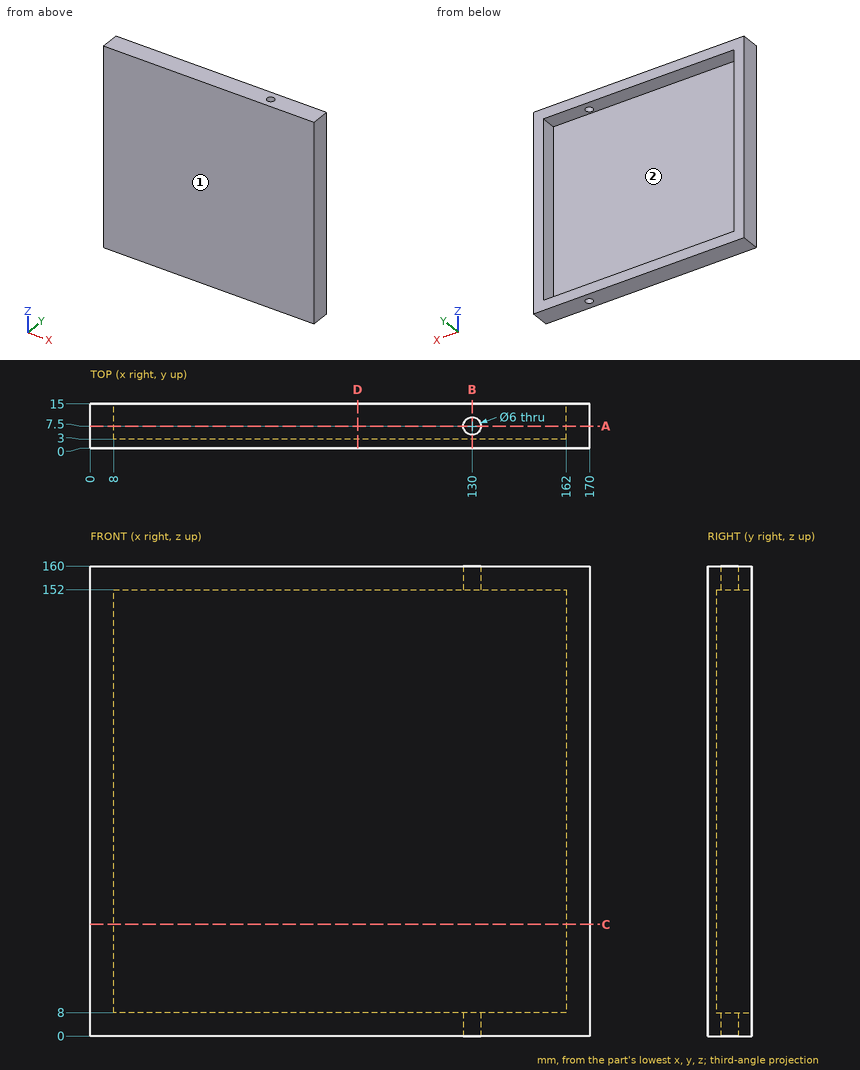
Design review of the part shown in the three views and the two pictorial views. Dimensions are in mm from the part's minimum x, y and z. Round coordinates to 2 decimals unless told otherwise and drop trailing zeros. Write each loop counter-clockwise with the first axis right and the second up, starting at its lowest first coordinate (ties: lowest second). Pieces come first, ordered by that corner, then holes. Notation, with made-up numbers: (71.5, 65.25) -> (112.5, 65.25) arc R17 cw to (112.5, 96.25) -> close; hole circle Ø3 at (-18.75, -23). An arc over 180 degrees is marked (long way). One line per question, with ' | ' between items. Start each with the question number.
1) Add section B-B (x = 130). Write out the cut boundary in (y, z).
2) Wall thickness on line 1 along Z through (x, y) = (89.5, 10.5); line 2 along X through (y, z) = (7.5, 155.25); line 3 along X through (y, z) = (9.75, 62): over which ranges is each line inside the solid? List them lowest first.
3) Add section C-C (z = 38). Write out the cut boundary in (x, y), and give its area (3 significant figures).
4) Mouldability with a two-part tool opening along Z and no side actions: class the marked faces 1 and 2 as +Z half, -Z half, draft (parallel to the pull), parting line (faces both ways), or undercut.
5) Add section D-D (x = 91). Write out the cut boundary in (y, z).
6) Add section A-A (y = 7.5). Write out the cut boundary in (x, z), and give its area (3 significant figures).
7) For pin 1 Ø5 at (x, z) = (90, 45) entering from +Y, flat-tipped, find the tip position at first contact; note if it passes through.
Reported:
1) outline: (0, 0) -> (4.5, 0) -> (4.5, 8) -> (3, 8) -> (3, 152) -> (4.5, 152) -> (4.5, 160) -> (0, 160) -> close; (10.5, 0) -> (15, 0) -> (15, 8) -> (10.5, 8) -> close; (10.5, 152) -> (15, 152) -> (15, 160) -> (10.5, 160) -> close
2) line 1: z = 0 to 8, 152 to 160 | line 2: x = 0 to 127, 133 to 170 | line 3: x = 0 to 8, 162 to 170
3) outline: (0, 0) -> (170, 0) -> (170, 15) -> (162, 15) -> (162, 3) -> (8, 3) -> (8, 15) -> (0, 15) -> close | area: 702 mm²
4) face 1: draft | face 2: undercut
5) outline: (0, 0) -> (15, 0) -> (15, 8) -> (3, 8) -> (3, 152) -> (15, 152) -> (15, 160) -> (0, 160) -> close
6) outline: (0, 0) -> (127, 0) -> (127, 8) -> (8, 8) -> (8, 152) -> (127, 152) -> (127, 160) -> (0, 160) -> close; (133, 0) -> (170, 0) -> (170, 160) -> (133, 160) -> (133, 152) -> (162, 152) -> (162, 8) -> (133, 8) -> close | area: 4,930 mm²
7) pin 1: stops at y = 3
